The model under review builds one solid part; all positions refer to its coordinate system, in mm. A direction names the side the tool comes from. Give positions to 0.01 mm unless a question says otherwise; leave off trailing zeros. Loops run counter-clockwise (first coordinate to the right, second up) from the corner with the lowest first, then second, coordinate; pieces in that order, holes last. Notation, with made-up numbers: (-19, 86.25) - (-12, 86.25) arc R15 ccw to (-12, 98.25) - close; hole circle Ø10 at (0.25, -29). An arc over 180 degrees is marked (long way). Answer as a JSON object with one key per item and string values.
from build123d import *

# Parameters (mm, degrees)
SKETCH1_R           = 3
BOSS_EXTRUDE2_DEPTH = 5
SKETCH2_R           = 10
SKETCH2_R_2         = 3
BOSS_EXTRUDE3_DEPTH = 7.5


# Read off the part's stored shape, not the designer's step: CSK for M3 Flat Head Machine Screw1
with BuildPart() as part:
    # Sketch1 → Boss-Extrude2 (new body)
    with BuildSketch(Plane.XY):
        with BuildLine():
            ThreePointArc((-19.550519413, 15.581309017), (-18.238129642, 12.880402273), (-16.110253623, 10.761580005))
            ThreePointArc((-16.110253623, 10.761580005), (-16.778376173, 9.687), (-17.374928481, 8.571098896))
            ThreePointArc((-17.374928481, 8.571098896), (-20.2738204, 9.354482451), (-23.269069139, 9.14059196))
            ThreePointArc((-23.269069139, 9.14059196), (-23.49231552, 8.550503583), (-23.700600368, 7.954969654))
            ThreePointArc((-23.700600368, 7.954969654), (-21.543592873, 5.865811255), (-18.819363584, 4.602546066))
            ThreePointArc((-18.819363584, 4.602546066), (-19.079665407, 3.364259794), (-19.258580553, 2.111622855))
            ThreePointArc((-19.258580553, 2.111622855), (-22.250580854, 1.856283171), (-24.992039135, 0.630856452))
            ThreePointArc((-24.992039135, 0.630856452), (-25, 0), (-24.992039135, -0.630856452))
            ThreePointArc((-24.992039135, -0.630856452), (-22.250580854, -1.856283171), (-19.258580553, -2.111622855))
            ThreePointArc((-19.258580553, -2.111622855), (-19.079665407, -3.364259794), (-18.819363584, -4.602546066))
            ThreePointArc((-18.819363584, -4.602546066), (-21.543592873, -5.865811255), (-23.700600368, -7.954969654))
            ThreePointArc((-23.700600368, -7.954969654), (-23.49231552, -8.550503583), (-23.269069139, -9.14059196))
            ThreePointArc((-23.269069139, -9.14059196), (-20.2738204, -9.354482451), (-17.374928481, -8.571098896))
            ThreePointArc((-17.374928481, -8.571098896), (-16.778376173, -9.687), (-16.110253623, -10.761580005))
            ThreePointArc((-16.110253623, -10.761580005), (-18.238129642, -12.880402273), (-19.550519413, -15.581309017))
            ThreePointArc((-19.550519413, -15.581309017), (-19.151111078, -16.069690242), (-18.739505991, -16.547837177))
            ThreePointArc((-18.739505991, -16.547837177), (-15.851737997, -15.724393089), (-13.395603607, -13.996773914))
            ThreePointArc((-13.395603607, -13.996773914), (-12.45336715, -14.841345041), (-11.458009312, -15.622608572))
            ThreePointArc((-11.458009312, -15.622608572), (-12.73287881, -18.341426683), (-13.042357282, -21.328312557))
            ThreePointArc((-13.042357282, -21.328312557), (-12.5, -21.650635095), (-11.949681854, -21.95916901))
            ThreePointArc((-11.949681854, -21.95916901), (-9.517702044, -20.197709854), (-7.800571241, -17.734231427))
            ThreePointArc((-7.800571241, -17.734231427), (-6.626298257, -18.205604835), (-5.423759977, -18.59931998))
            ThreePointArc((-5.423759977, -18.59931998), (-5.691854876, -21.590204344), (-4.961094377, -24.502806831))
            ThreePointArc((-4.961094377, -24.502806831), (-4.341204442, -24.620193825), (-3.718549727, -24.721900977))
            ThreePointArc((-3.718549727, -24.721900977), (-2.035690758, -22.234884724), (-1.264674858, -19.332678901))
            ThreePointArc((-1.264674858, -19.332678901), (0, -19.374), (1.264674858, -19.332678901))
            ThreePointArc((1.264674858, -19.332678901), (2.035690758, -22.234884724), (3.718549727, -24.721900977))
            ThreePointArc((3.718549727, -24.721900977), (4.341204442, -24.620193825), (4.961094377, -24.502806831))
            ThreePointArc((4.961094377, -24.502806831), (5.691854876, -21.590204344), (5.423759977, -18.59931998))
            ThreePointArc((5.423759977, -18.59931998), (6.626298257, -18.205604835), (7.800571241, -17.734231427))
            ThreePointArc((7.800571241, -17.734231427), (9.517702044, -20.197709854), (11.949681854, -21.95916901))
            ThreePointArc((11.949681854, -21.95916901), (12.5, -21.650635095), (13.042357282, -21.328312557))
            ThreePointArc((13.042357282, -21.328312557), (12.73287881, -18.341426683), (11.458009312, -15.622608572))
            ThreePointArc((11.458009312, -15.622608572), (12.45336715, -14.841345041), (13.395603607, -13.996773914))
            ThreePointArc((13.395603607, -13.996773914), (15.851737997, -15.724393089), (18.739505991, -16.547837177))
            ThreePointArc((18.739505991, -16.547837177), (19.151111078, -16.069690242), (19.550519413, -15.581309017))
            ThreePointArc((19.550519413, -15.581309017), (18.238129642, -12.880402273), (16.110253623, -10.761580005))
            ThreePointArc((16.110253623, -10.761580005), (16.778376173, -9.687), (17.374928481, -8.571098896))
            ThreePointArc((17.374928481, -8.571098896), (20.2738204, -9.354482451), (23.269069139, -9.14059196))
            ThreePointArc((23.269069139, -9.14059196), (23.49231552, -8.550503583), (23.700600368, -7.954969654))
            ThreePointArc((23.700600368, -7.954969654), (21.543592873, -5.865811255), (18.819363584, -4.602546066))
            ThreePointArc((18.819363584, -4.602546066), (19.079665407, -3.364259794), (19.258580553, -2.111622855))
            ThreePointArc((19.258580553, -2.111622855), (22.250580854, -1.856283171), (24.992039135, -0.630856452))
            ThreePointArc((24.992039135, -0.630856452), (25, 0), (24.992039135, 0.630856452))
            ThreePointArc((24.992039135, 0.630856452), (22.250580854, 1.856283171), (19.258580553, 2.111622855))
            ThreePointArc((19.258580553, 2.111622855), (19.079665407, 3.364259794), (18.819363584, 4.602546066))
            ThreePointArc((18.819363584, 4.602546066), (21.543592873, 5.865811255), (23.700600368, 7.954969654))
            ThreePointArc((23.700600368, 7.954969654), (23.49231552, 8.550503583), (23.269069139, 9.14059196))
            ThreePointArc((23.269069139, 9.14059196), (20.2738204, 9.354482451), (17.374928481, 8.571098896))
            ThreePointArc((17.374928481, 8.571098896), (16.778376173, 9.687), (16.110253623, 10.761580005))
            ThreePointArc((16.110253623, 10.761580005), (18.238129642, 12.880402273), (19.550519413, 15.581309017))
            ThreePointArc((19.550519413, 15.581309017), (19.151111078, 16.069690242), (18.739505991, 16.547837177))
            ThreePointArc((18.739505991, 16.547837177), (15.851737997, 15.724393089), (13.395603607, 13.996773914))
            ThreePointArc((13.395603607, 13.996773914), (12.45336715, 14.841345041), (11.458009312, 15.622608572))
            ThreePointArc((11.458009312, 15.622608572), (12.73287881, 18.341426683), (13.042357282, 21.328312557))
            ThreePointArc((13.042357282, 21.328312557), (12.5, 21.650635095), (11.949681854, 21.95916901))
            ThreePointArc((11.949681854, 21.95916901), (9.517702044, 20.197709854), (7.800571241, 17.734231427))
            ThreePointArc((7.800571241, 17.734231427), (6.626298257, 18.205604835), (5.423759977, 18.59931998))
            ThreePointArc((5.423759977, 18.59931998), (5.691854876, 21.590204344), (4.961094377, 24.502806831))
            ThreePointArc((4.961094377, 24.502806831), (4.341204442, 24.620193825), (3.718549727, 24.721900977))
            ThreePointArc((3.718549727, 24.721900977), (2.035690758, 22.234884724), (1.264674858, 19.332678901))
            ThreePointArc((1.264674858, 19.332678901), (0, 19.374), (-1.264674858, 19.332678901))
            ThreePointArc((-1.264674858, 19.332678901), (-2.035690758, 22.234884724), (-3.718549727, 24.721900977))
            ThreePointArc((-3.718549727, 24.721900977), (-4.341204442, 24.620193825), (-4.961094377, 24.502806831))
            ThreePointArc((-4.961094377, 24.502806831), (-5.691854876, 21.590204344), (-5.423759977, 18.59931998))
            ThreePointArc((-5.423759977, 18.59931998), (-6.626298257, 18.205604835), (-7.800571241, 17.734231427))
            ThreePointArc((-7.800571241, 17.734231427), (-9.517702044, 20.197709854), (-11.949681854, 21.95916901))
            ThreePointArc((-11.949681854, 21.95916901), (-12.5, 21.650635095), (-13.042357282, 21.328312557))
            ThreePointArc((-13.042357282, 21.328312557), (-12.73287881, 18.341426683), (-11.458009312, 15.622608572))
            ThreePointArc((-11.458009312, 15.622608572), (-12.45336715, 14.841345041), (-13.395603607, 13.996773914))
            ThreePointArc((-13.395603607, 13.996773914), (-15.851737997, 15.724393089), (-18.739505991, 16.547837177))
            ThreePointArc((-18.739505991, 16.547837177), (-19.151111078, 16.069690242), (-19.550519413, 15.581309017))
        make_face()
        Circle(SKETCH1_R, mode=Mode.SUBTRACT)
    extrude(amount=BOSS_EXTRUDE2_DEPTH)

    # Sketch2 → Boss-Extrude3 (add)
    with BuildSketch(Plane.XY.offset(5)):
        Circle(SKETCH2_R)
        Circle(SKETCH2_R_2, mode=Mode.SUBTRACT)
    extrude(amount=BOSS_EXTRUDE3_DEPTH)

    # CSK for M3 Flat Head Machine Screw1 outl → CSK for M3 Flat Head Machine Screw1 (revolve, cut)
    with BuildSketch(Plane(origin=(0, 0, 8.675124241), x_dir=(0.9261648448832729, -0.37711892037173506, 0), z_dir=(0, 0, 1))):
        Polygon((3.150067458, -10.000067458), (1.7, -8.55), (1.7, -3), (1.247536555, -2.728132535), (0, -2.728132535), (0, -10.000067458), align=None)
    revolve(axis=Axis((0, 0, 8.675124241), (0.37711892037173506, 0.9261648448832729, 0)), mode=Mode.SUBTRACT)


solid = part.part
Q1. Consider section A-A, the plane y = 0. State the section outline as (x, z) points, plus the area to 3 significant figures.
Results:
{"outline": "(-25, 0) - (-3, 0) - (-3, 12.5) - (-10, 12.5) - (-10, 5) - (-25, 5) - close; (3, 0) - (25, 0) - (25, 5) - (10, 5) - (10, 12.5) - (3, 12.5) - close", "area": "325 mm^2"}
Q2. For faces 4 (the face through (-12.508, -21.646, 2.465)), 5 (the face through (-21.58, 5.89, 2.46)), 6 (the face through (15.89, 15.742, 2.465)), 7 (the face through (-4.333, 24.622, 2.465)), 8 (the face through (-12.5, -14.8, 2.5)), list the 3-axis set-ups (+Z, -Z, +X, -X, +Y, -Y) from which the entire face can be reached by the end or side of a thin tool; tool diameter is ignored.
Results:
{"face 4": "+Z, -Z, -X, -Y", "face 5": "+Z, -Z, -X", "face 6": "+Z, -Z, +Y", "face 7": "+Z, -Z, -X, +Y", "face 8": "+Z, -Z"}
Q3. Clearance check with flat-ended pins moving along their axes: pin 1 Ø5 at (x, y) = (15, -11.5) entering from +Z; pin 2 Ø2 at (x, y) = (-20, 13) entering from +Z; pin 3 Ø5 at (y, z) = (-16.5, 4) entering from +X; pin 4 Ø4 at (y, z) = (-8, 5) entering from -X. State where each tip first meets the part, or that it passes through.
Results:
{"pin 1": "stops at z = 5", "pin 2": "passes through", "pin 3": "stops at x = 19.55", "pin 4": "stops at x = -23.7"}
Q4. The part is to be moulded in two halves that separate along Y. For faces 1 (the face through (5.69, -21.63, 2.46)), 2 (the face through (12.508, 21.646, 2.465)), 3 (the face through (0, -5, 0)), say which applies: +Y half, -Y half, draft (parallel to the pull), parting line (faces both ways), or undercut.
Results:
{"face 1": "undercut", "face 2": "+Y half", "face 3": "draft"}
Q5. To check wall thickness, follow probe 1 along Y at (x, z) = (0, 4.25); probe 2 along Z at (x, y) = (6, -10.5); probe 3 along Y at (x, z) = (0, 6.75). State the ranges of each line that lie inside material, in increasing order. Write a range as [from, to].
Results:
{"probe 1": "y = [-19.37, -3], [3, 19.37]", "probe 2": "z = [0, 5]", "probe 3": "y = [-10, -3], [3, 10]"}
